from build123d import *

# Parameters (mm, degrees)
SKETCH1_R           = 2.5
BOSS_EXTRUDE1_DEPTH = 2


with BuildPart() as part:
    # Sketch1 → Boss-Extrude1 (new body)
    with BuildSketch(Plane(origin=(0, 0, 0), x_dir=(1, 0, 0), z_dir=(0, 1, 0))):
        with BuildLine():
            Line((63.73099869, -373.254460076), (114.596265016, -294.778975996))
            Line((114.596265016, -294.778975996), (114.596265016, -462.608083148))
            Line((114.596265016, -462.608083148), (63.73099869, -384.132599068))
            ThreePointArc((63.73099869, -384.132599068), (62.122454047, -378.693529572), (63.73099869, -373.254460076))
        make_face()
        with Locations((72.122454047, -378.693529572)):
            Circle(SKETCH1_R, mode=Mode.SUBTRACT)
        with Locations((93.878732031, -345.127708141)):
            Circle(SKETCH1_R, mode=Mode.SUBTRACT)
        with Locations((104.756871022, -328.344797426)):
            Circle(SKETCH1_R, mode=Mode.SUBTRACT)
        with Locations((93.878732031, -412.259351002)):
            Circle(SKETCH1_R, mode=Mode.SUBTRACT)
        with Locations((104.756871022, -429.042261718)):
            Circle(SKETCH1_R, mode=Mode.SUBTRACT)
    extrude(amount=BOSS_EXTRUDE1_DEPTH)


solid = part.part
Input: part model. Units: mm. Frame: model coordinates. Coordinates: 2 decimals unless noted, no trailing zeros. Order: outer loops, then holes, each group sorted by start corner. A loop starts at its lowest first (then second) coordinate and runs counter-clockwise, first axis right, second up. Notation, with made-up numbers: M 3.5,-7 L 32.5,-7 A15 ccw 32.5,20 Z; hole C 64,-24 d3. An arc over 180 degrees is marked long. Answer as CSV lines item,"result".
1. First-contact query: P1, Ø4, axis at x = 104.76, z = 429.04, coming from the -Y side; P2, Ø1, axis at y = 1, z = 367.5, coming from the -X side. Flat tips, straight axial feed; report the tip coordinate or a pass-through.
Reported:
P1,"through"
P2,"x = 67.14"
2. Section D-D (x = 80). Return the cut outline in (y, z).
Reported:
outline,"M 0,348.15 L 2,348.15 L 2,409.23 L 0,409.23 Z"
3. Section C-C (z = 445.5). Return the cut outline in (x, y), then the cut area to 3 significant figures.
Reported:
outline,"M 103.51,0 L 114.6,0 L 114.6,2 L 103.51,2 Z"
area,"22.2 mm2"
4. Section B-B (y = 1.35). Return the cut outline in (x, z).
Reported:
outline,"M 63.73,373.25 L 114.6,294.78 L 114.6,462.61 L 63.73,384.13 A10 ccw Z; hole C 72.12,378.69 d5; hole C 93.88,345.13 d5; hole C 93.88,412.26 d5; hole C 104.76,328.34 d5; hole C 104.76,429.04 d5"
5. Material intervals for line 1 (Z direction, x = 96, y = 0.45); line 2 (Z direction, x = 107, y = 0.8); line 3 (Z direction, x = 72, y = 0.2), sorted ascending. Write a range as from..to.
Reported:
line 1,"323.47..343.8, 346.45..410.94, 413.58..433.92"
line 2,"306.5..327.24, 329.45..427.94, 430.15..450.89"
line 3,"360.5..376.2, 381.19..396.89"
6. Section A-A (x = 73). Return the cut outline in (y, z), then the cut area to 3 significant figures.
Reported:
outline,"M 0,358.95 L 2,358.95 L 2,376.35 L 0,376.35 Z; M 0,381.03 L 2,381.03 L 2,398.43 L 0,398.43 Z"
area,"69.6 mm2"
7. Pull-direction query (X, two-part tool) for faces 1 (the flat face through (89.52, 0.99, 423.92)), 2 (the flat face through (100, 2, 378)), 3 (the cylindrical face through (95.22, 0.99, 410.15)); classes: released by +X, released by -X, zero draft, split by the parting line, or undercut.
Reported:
face 1,"released by -X"
face 2,"zero draft"
face 3,"undercut"
